from build123d import *

# Parameters (mm, degrees)
ESQUISSE1_W                  = 57.5
ESQUISSE1_H                  = 32
BOSS_EXTRU_1_DEPTH           = 9
ESQUISSE2_W                  = 24.25
ESQUISSE2_H                  = 32
ESQUISSE2_W_2                = 24
ESQUISSE2_W_3                = 5.25
ENL_V_MAT_EXTRU_1_DEPTH      = 7.75
ESQUISSE3_R                  = 1.55
ENL_V_MAT_EXTRU_2_DEPTH      = 34.5
CONG_1_R                     = 3
CONG_2_R                     = 2
ESQUISSE10_R                 = 3
BOSS_EXTRU_2_DEPTH           = 2
ESQUISSE9_R                  = 1.5
ENL_V_MAT_EXTRU_3_DEPTH      = 8.75
ENL_V_MAT_EXTRU_3_DEPTH_BACK = 2.25


with BuildPart() as part:
    # Esquisse1 → Boss.-Extru.1 (new body)
    with BuildSketch(Plane.XY):
        with Locations((28.75, 16)):
            Rectangle(ESQUISSE1_W, ESQUISSE1_H)
    extrude(amount=BOSS_EXTRU_1_DEPTH)

    # Esquisse2 → Enlèv. mat.-Extru.1 (cut)
    with BuildSketch(Plane(origin=(0, 0, 0), x_dir=(-1, 0, 0), z_dir=(0, 0, -1))):
        with Locations((-12.125, 16)):
            Rectangle(ESQUISSE2_W, ESQUISSE2_H)
        with Locations((-45.5, 16)):
            Rectangle(ESQUISSE2_W_2, ESQUISSE2_H)
        with Locations((-28.875, 16)):
            Rectangle(ESQUISSE2_W_3, ESQUISSE2_H)
    extrude(amount=-ENL_V_MAT_EXTRU_1_DEPTH, mode=Mode.SUBTRACT)

    # Esquisse3 → Enlèv. mat.-Extru.2 (cut, through all)
    with BuildSketch(Plane(origin=(33.5, 0, 0), x_dir=(0, 0, -1), z_dir=(1, 0, 0))):
        with Locations((-3.5, 10)):
            Circle(ESQUISSE3_R)
        with Locations((-3.5, 20)):
            Circle(ESQUISSE3_R)
    extrude(amount=-ENL_V_MAT_EXTRU_2_DEPTH, mode=Mode.SUBTRACT)

    # Congé1
    cong_1_edges = [part.edges().sort_by_distance(p)[0] for p in [
        (0, 32, 8.375),
        (57.5, 32, 8.375),
        (57.5, 0, 8.375),
        (0, 0, 8.375),
    ]]
    fillet(cong_1_edges, radius=CONG_1_R)

    # Congé2
    cong_2_edges = [part.edges().sort_by_distance(p)[0] for p in [
        (32.5, 32, 0),
        (25.25, 32, 0),
        (25.25, 0, 0),
        (32.5, 0, 0),
    ]]
    fillet(cong_2_edges, radius=CONG_2_R)

    # Esquisse10 → Boss.-Extru.2 (add)
    with BuildSketch(Plane(origin=(0, 0, 7.75), x_dir=(-1, 0, 0), z_dir=(0, 0, -1))):
        with Locations((-54.5, 28.5)):
            Circle(ESQUISSE10_R)
        with Locations((-54.5, 3.5)):
            Circle(ESQUISSE10_R)
        with Locations((-3, 3.5)):
            Circle(ESQUISSE10_R)
        with Locations((-3, 28.5)):
            Circle(ESQUISSE10_R)
    extrude(amount=BOSS_EXTRU_2_DEPTH)

    # Esquisse9 → Enlèv. mat.-Extru.3 (cut, two sides)
    with BuildSketch(Plane(origin=(0, 0, 7.75), x_dir=(-1, 0, 0), z_dir=(0, 0, -1))) as enl_v_mat_extru_3_sk:
        with Locations((-54.5, 28.5)):
            Circle(ESQUISSE9_R)
        with Locations((-3, 28.5)):
            Circle(ESQUISSE9_R)
        with Locations((-3, 3.5)):
            Circle(ESQUISSE9_R)
        with Locations((-54.5, 3.5)):
            Circle(ESQUISSE9_R)
    extrude(amount=ENL_V_MAT_EXTRU_3_DEPTH, mode=Mode.SUBTRACT)
    extrude(enl_v_mat_extru_3_sk.sketch, amount=-ENL_V_MAT_EXTRU_3_DEPTH_BACK, mode=Mode.SUBTRACT)


solid = part.part
Verification items for the finished model (mm, model axes). A direction names the side the tool comes from. Give positions to 0.01 mm unless a question says otherwise; leave off trailing zeros. Loops run counter-clockwise (first coordinate to the right, second up) from the corner with the lowest first, then second, coordinate; pieces in that order, holes last.
1) Draft check along Y on faces 4 (the flat face through (32, 16, 0)), 5 (the cylindrical face through (25.26, 31.43, 0.6)), 6 (the cylindrical face through (32.51, 9.06, 4.73)). Enter one of: pulls with the +Y half, pulls with the -Y half, needs draft (parallel to the pull), parting line crosses it, or undercut.
2) Sectioned sample at C-C, the plane y = 16. Enter the section's corners in (x, z), then the cut area to 3 significant figures.
3) Sectioned sample at B-B, the plane z = 3.5. Enter the section's corners in (x, y).
4) Thickness scan on line 1 along Y through (x, z) = (32.95, 3.5); line 2 along Y through (x, z) = (54.5, 7.3); line 3 along X through (y, z) = (16, 4.25). Record the ranges inside material, lowest first.
5) Set-up check for faces 1 (the flat face through (2, 5, 5.75)), 2 (the flat face through (31.5, 16, 4)), 3 (the cylindrical face through (5.21, 5.53, 6.76)): record each of +Z, -Z, +X, -X, +Y, -Y from which the full face is reachable in a straight line by a thin tool's end or side.
6) Depth check by flat-ended pin: pin 1 Ø3 at (y, z) = (10, 3.5) entering from -X; pin 2 Ø4 at (y, z) = (22, 5.5) entering from -X; pin 3 Ø2.5 at (x, y) = (29.5, 12.5) entering from -Z; pin 4 Ø6.5 at (x, y) = (55, 28) entering from -Z. Enter the tip coordinate at first touch or a pass-through.
7) Sectioned sample at A-A, the plane y = 20. Enter the section's corners in (x, z), then the cut area to 3 significant figures.
8) Sectioned sample at D-D, the plane z = 1. Enter the section's corners in (x, y).
Answers:
1. face 4: needs draft
1. face 5: pulls with the +Y half
1. face 6: undercut
2. outline: (0, 7.75) - (24.25, 7.75) - (24.25, 0) - (26.25, 0) - (26.25, 7.75) - (31.5, 7.75) - (31.5, 0) - (33.5, 0) - (33.5, 7.75) - (57.5, 7.75) - (57.5, 9) - (0, 9) - close
2. area: 103 mm2
3. outline: (24.25, 0) - (26.25, 0) - (26.25, 8.45) - (24.25, 8.45) - close; (24.25, 11.55) - (26.25, 11.55) - (26.25, 18.45) - (24.25, 18.45) - close; (24.25, 21.55) - (26.25, 21.55) - (26.25, 32) - (24.25, 32) - close; (31.5, 0) - (33.5, 0) - (33.5, 8.45) - (31.5, 8.45) - close; (31.5, 11.55) - (33.5, 11.55) - (33.5, 18.45) - (31.5, 18.45) - close; (31.5, 21.55) - (33.5, 21.55) - (33.5, 32) - (31.5, 32) - close
4. line 1: y = 0 to 8.45, 11.55 to 18.45, 21.55 to 32
4. line 2: y = 0.5 to 2, 5 to 6.5, 25.5 to 27, 30 to 31.5
4. line 3: x = 24.25 to 26.25, 31.5 to 33.5
5. face 1: -Z, -X, +Y, -Y
5. face 2: -Z, +Y, -Y
5. face 3: -Z
6. pin 1: passes through
6. pin 2: stops at x = 24.25
6. pin 3: stops at z = 7.75
6. pin 4: stops at z = 5.75
7. outline: (0, 7.75) - (24.25, 7.75) - (24.25, 5.05) - (26.25, 5.05) - (26.25, 7.75) - (31.5, 7.75) - (31.5, 5.05) - (33.5, 5.05) - (33.5, 7.75) - (57.5, 7.75) - (57.5, 9) - (0, 9) - close; (24.25, 0) - (26.25, 0) - (26.25, 1.95) - (24.25, 1.95) - close; (31.5, 0) - (33.5, 0) - (33.5, 1.95) - (31.5, 1.95) - close
7. area: 90.5 mm2
8. outline: (24.25, 0.27) - (26.25, 0.27) - (26.25, 31.73) - (24.25, 31.73) - close; (31.5, 0.27) - (33.5, 0.27) - (33.5, 31.73) - (31.5, 31.73) - close
